The listing builds one solid part. Answer for the finished solid, in the listing's coordinates (mm). Face numbers are marked on the shaded views. A direction names the side the tool comes from. Give positions to 0.01 mm unless a question says otherwise; leave off trailing zeros. Order: outer loops, then holes, each group sorted by start corner. A loop starts at its lowest first (then second) coordinate and runs counter-clockwise, first axis right, second up. Notation, with made-up numbers: (36, -8) - (46, -8) arc R21 cw to (46, 31) - close; hole circle Ø2 at (49.5, 19.5). An arc over 180 degrees is marked (long way). Answer as CSV lines item,"result". Start each with the question number.
1. Section A-A on x = -113.5 is taken. Give the vertices of the cut face in (y, z), and give its area (3 significant figures).
2. Section B-B on y = 34 is taken. Give the vertices of the cut face in (x, z), and give its area (3 significant figures).
3. Which of the six approach directions +Z, -Z, +X, -X, +Y, -Y give full straight-line access (tool end or side, diameter ignored) to the marked faces 1 and 2?
4. Section D-D on z = 52.5 is taken. Give the vertices of the cut face in (x, y).
5. Section C-C on x = 197 is taken. Give the vertices of the cut face in (y, z).
6. Flat-ended cylindrical pins translate along their axes: pin 1 (10 mm diameter, centred on x = -59, y = 33.5, fed in from -Z); pin 2 (1.5 mm diameter, centred on x = 148.5, z = 124, fed in from +Y); pin 3 (12 mm diameter, centred on x = 74, z = 58, fed in from -Y). Find the tip coordinate at first contact, or state that the pin passes through.
7. Consider line 1 along Z through (x, y) = (182, 33.5); line 2 along Z through (x, y) = (127, 19); line 3 along Y through (x, z) = (33.5, 64). Determine where each line is inside the solid, lowest interval first. Write a range as [from, to].
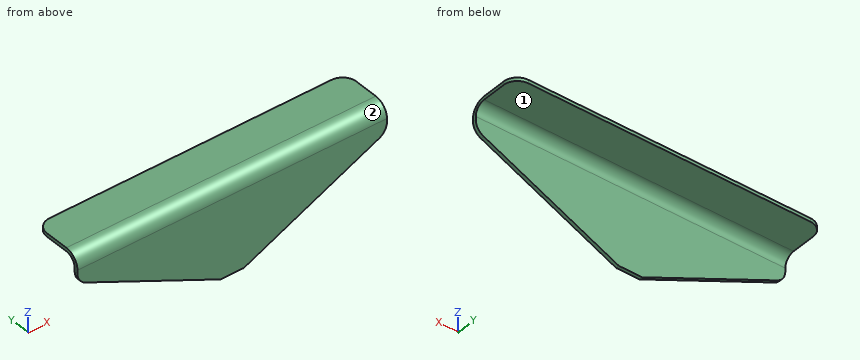
from build123d import *

# Parameters (mm, degrees)
F2_DEPTH = 250
F3_DEPTH = 100
F4_R     = 20


with BuildPart() as f2:
    # F1 (on Right) → F2 (new body)
    with BuildSketch(Plane.YZ):
        with BuildLine():
            Line((0, 154.855098), (0, 42.036165))
            Line((0, 42.036165), (5, 42.036165))
            Line((5, 42.036165), (5, 154.855098))
            ThreePointArc((5, 154.855098), (9.393398, 165.4617), (20, 169.855098))
            Line((20, 169.855098), (75, 169.855098))
            Line((75, 169.855098), (75, 174.855098))
            Line((75, 174.855098), (20, 174.855098))
            ThreePointArc((20, 174.855098), (5.857864, 168.997234), (0, 154.855098))
        make_face()
    extrude(amount=F2_DEPTH)

    # F0 (on Front) → F3 (cut)
    with BuildSketch(Plane.XZ):
        with BuildLine():
            Line((291.145295, 178.066522), (224.921591, 175.062526))
            Line((224.921591, 175.062526), (224.999902, 150.062649))
            ThreePointArc((224.999902, 150.062649), (221.844029, 139.216741), (213.315195, 131.81051))
            Line((213.315195, 131.81051), (61.684805, 62.493761))
            Line((61.684805, 62.493761), (-75.020296, 0))
            Line((-75.020296, 0), (292.977542, 0))
            Line((292.977542, 0), (291.145295, 62.493761))
            Line((291.145295, 62.493761), (291.145295, 178.066522))
        make_face()
    extrude(amount=-F3_DEPTH, mode=Mode.SUBTRACT)

    # F4
    f4_edges = [f2.edges().sort_by_distance(p)[0] for p in [
        (224.930072, 75, 172.355098),
    ]]
    fillet(f4_edges, radius=F4_R)

    # F5: F2 across plane


with BuildPart() as f2_1:
    add(f2.part)
    add(f2.part.mirror(Plane.YZ))


solid = f2_1.part
Checks:
1,outline,"(0, 86.18) - (5, 86.18) - (5, 154.86) arc R15 cw to (20, 169.86) - (75, 169.86) - (75, 174.86) - (20, 174.86) arc R20 ccw to (0, 154.86) - close"
1,area,"756 mm²"
2,outline,"(-224.94, 169.86) - (224.94, 169.86) - (224.92, 174.86) - (-224.92, 174.86) - close"
2,area,"2,250 mm²"
3,face 1,"-Z, +X, -X, +Y"
3,face 2,"+Z, +X, -X, -Y"
4,outline,"(-39.82, 0) - (39.82, 0) - (39.82, 5) - (-39.82, 5) - close"
5,outline,"(0, 124.35) - (5, 124.35) - (5, 154.86) arc R15 cw to (20, 169.86) - (75, 169.86) - (75, 174.86) - (20, 174.86) arc R20 ccw to (0, 154.86) - close"
6,pin 1,"stops at z = 169.86"
6,pin 2,"stops at y = 5"
6,pin 3,"passes through"
7,line 1,"z = [169.86, 174.86]"
7,line 2,"z = [169.82, 174.83]"
7,line 3,"y = [0, 5]"
